Check sheet for the modelled part. Datum: model origin and axes. Units: mm. A direction names the side the tool comes from. Give positions to 0.01 mm unless a question says otherwise; leave off trailing zeros. Loops run counter-clockwise (first coordinate to the right, second up) from the corner with the lowest first, then second, coordinate; pieces in that order, holes last. Notation, with made-up numbers: (72, 40.5) -> (81, 40.5) arc R24 cw to (81, 61.5) -> close; hole circle Ø4 at (17, 33). An arc over 180 degrees is marked (long way). Write each question's results on one line, items separated by ' | '. Start each with the question number.
Item 1: Cross-section at A-A on y = 8.5. Enter the section's corners in (x, z).
Item 2: Mould release check, pull along X, two halves, no side actions. Record for faces 1 (the face through (43.6, 3, -25.9)), 2 (the face through (38.7, 1.2, -24.6)), 3 (the face through (42.15, 14, 0)): pulls with the +X half, pulls with the -X half, needs draft (parallel to the pull), parting line crosses it, or undercut.
Item 3: Access from +Z, -Z, +X, -X, +Y, -Y to the whole of each face (thin tool, end or side, straight path). Record for faces 4 (the face through (0, 13, 0)), 5 (the face through (43, 3, 26)), 6 (the face through (-36, 6, 0)), 7 (the face through (-38.56, 2.11, -28.46)).
Item 4: Scan lines: line 1 along Z through (x, y) = (40, 0.5); line 2 along X through (y, z) = (0.6, 26); line 3 along X through (y, z) = (14.7, 24.5). Record each from-to range of solid material in increasing order.
Item 5: Gauge pin test, flat ends, axial feed: pin 1 Ø1.3 at (x, z) = (36.5, -1) entering from -Y; pin 2 Ø8 at (x, z) = (-7, 2.5) entering from -Y; pin 3 Ø0.8 at (y, z) = (14, 25) entering from -X. Record the tip position at first contact, or that the pin passes through.
Item 6: Cross-section at B-B on z = 4.5. Enter the section's corners in (x, y).
from build123d import *

# Parameters (mm, degrees)
EXTRUDE_1_DEPTH          = 31
CUT_EXTRUDE_1_DEPTH      = 56.874860179
CUT_EXTRUDE_1_DEPTH_BACK = 56.874860179
SKETCH_2_W               = 42
SKETCH_2_H               = 12
CUT_EXTRUDE_3_REACH      = 57.875
SKETCH_3_R               = 1.75
SKETCH_5_R               = 1.6
CUT_EXTRUDE_5_DEPTH      = 5
CUT_EXTRUDE_8_DEPTH      = 1.6
FILLET_1_R               = 1
FILLET_7_R               = 2
CUT_EXTRUDE_9_DEPTH      = 1.8
FILLET_5_R               = 0.5
FILLET_8_R               = 1


with BuildPart() as part:
    # 草圖1 → 填料-伸長1 (new, symmetric)
    with BuildSketch(Plane.XY):
        Polygon((-44, 0), (-44, 3), (-37.15, 3), (-37.15, 13), (-42.85, 13), (-42.85, 15), (42.15, 15), (42.15, 13), (37.15, 13), (37.15, 3), (44, 3), (44, 0), (35.5, 0), (35.5, 13), (-35.5, 13), (-35.5, 0), align=None)
    extrude(amount=EXTRUDE_1_DEPTH, both=True)

    # 草圖2 → 除料-伸長1 (cut, two sides: drawn at the far end of the back side and taken through both)
    with BuildSketch(Plane(origin=(0, 0, 0), x_dir=(0, 0, -1), z_dir=(1, 0, 0)).offset(-CUT_EXTRUDE_1_DEPTH_BACK)):
        Rectangle(SKETCH_2_W, SKETCH_2_H)
    extrude(amount=CUT_EXTRUDE_1_DEPTH + CUT_EXTRUDE_1_DEPTH_BACK, mode=Mode.SUBTRACT)

    # 草圖3 → 除料-伸長3 (cut, up to next)
    with BuildSketch(Plane(origin=(0, 0, 0), x_dir=(1, 0, 0), z_dir=(0, 1, 0)), mode=Mode.PRIVATE) as cut_extrude_3_sk1:
        with Locations(Location((-40, 26, 0), (0, 0, 90))):
            Circle(SKETCH_3_R)
    cut_extrude_3_tool1 = extrude(cut_extrude_3_sk1.sketch, amount=CUT_EXTRUDE_3_REACH, mode=Mode.PRIVATE) & part.part
    # 草圖3 → 除料-伸長3 (cut, up to next)
    with BuildSketch(Plane(origin=(0, 0, 0), x_dir=(1, 0, 0), z_dir=(0, 1, 0)), mode=Mode.PRIVATE) as cut_extrude_3_sk2:
        with Locations(Location((40, 26, 0), (0, 0, 90))):
            Circle(SKETCH_3_R)
    cut_extrude_3_tool2 = extrude(cut_extrude_3_sk2.sketch, amount=CUT_EXTRUDE_3_REACH, mode=Mode.PRIVATE) & part.part
    # 草圖3 → 除料-伸長3 (cut, up to next)
    with BuildSketch(Plane(origin=(0, 0, 0), x_dir=(1, 0, 0), z_dir=(0, 1, 0)), mode=Mode.PRIVATE) as cut_extrude_3_sk3:
        with Locations(Location((40, -26, 0), (0, 0, 90))):
            Circle(SKETCH_3_R)
    cut_extrude_3_tool3 = extrude(cut_extrude_3_sk3.sketch, amount=CUT_EXTRUDE_3_REACH, mode=Mode.PRIVATE) & part.part
    # 草圖3 → 除料-伸長3 (cut, up to next)
    with BuildSketch(Plane(origin=(0, 0, 0), x_dir=(1, 0, 0), z_dir=(0, 1, 0)), mode=Mode.PRIVATE) as cut_extrude_3_sk4:
        with Locations(Location((-40, -26, 0), (0, 0, 90))):
            Circle(SKETCH_3_R)
    cut_extrude_3_tool4 = extrude(cut_extrude_3_sk4.sketch, amount=CUT_EXTRUDE_3_REACH, mode=Mode.PRIVATE) & part.part
    add(cut_extrude_3_tool1.solids().sort_by_distance((-40, 0, -26))[0], mode=Mode.SUBTRACT)
    add(cut_extrude_3_tool2.solids().sort_by_distance((40, 0, -26))[0], mode=Mode.SUBTRACT)
    add(cut_extrude_3_tool3.solids().sort_by_distance((40, 0, 26))[0], mode=Mode.SUBTRACT)
    add(cut_extrude_3_tool4.solids().sort_by_distance((-40, 0, 26))[0], mode=Mode.SUBTRACT)

    # 草圖5 → 除料-伸長5 (cut)
    with BuildSketch(Plane(origin=(0, 15, 0), x_dir=(1, 0, 0), z_dir=(0, 1, 0))):
        with Locations(Location((-39.85, 24.5, 0), (0, 0, 270))):
            Circle(SKETCH_5_R)
        with Locations(Location((-39.85, -24.5, 0), (0, 0, 270))):
            Circle(SKETCH_5_R)
        with Locations(Location((18.15, 24.5, 0), (0, 0, 270))):
            Circle(SKETCH_5_R)
        with Locations(Location((18.15, -24.5, 0), (0, 0, 270))):
            Circle(SKETCH_5_R)
    extrude(amount=-CUT_EXTRUDE_5_DEPTH, mode=Mode.SUBTRACT)

    # 草圖17 → 除料-伸長8 (cut)
    with BuildSketch(Plane.XZ.offset(-13)):
        Polygon((20.75, 22.9988893), (20.75, 26.0011107), (18.15, 27.5022214), (15.55, 26.0011107), (15.55, 22.9988893), (18.15, 21.4977786), align=None)
        Polygon((20.75, -26.0011107), (20.75, -22.9988893), (18.15, -21.4977786), (15.55, -22.9988893), (15.55, -26.0011107), (18.15, -27.5022214), align=None)
        Polygon((-39.85, 21.4977786), (-37.25, 22.9988893), (-37.25, 26.0011107), (-39.85, 27.5022214), (-42.45, 26.0011107), (-42.45, 22.9988893), align=None)
        Polygon((-39.85, -27.5022214), (-37.25, -26.0011107), (-37.25, -22.9988893), (-39.85, -21.4977786), (-42.45, -22.9988893), (-42.45, -26.0011107), align=None)
    extrude(amount=-CUT_EXTRUDE_8_DEPTH, mode=Mode.SUBTRACT)

    # 圓角1
    fillet_1_edges = [part.edges().sort_by_distance(p)[0] for p in [
        (-44, 1.5, -31),
        (-42.85, 14, -31),
        (42.15, 14, -31),
        (44, 1.5, -31),
        (44, 1.5, 31),
        (42.15, 14, 31),
        (-44, 1.5, 21),
        (-44, 1.5, -21),
        (-42.85, 14, 31),
        (44, 1.5, -21),
        (44, 1.5, 21),
        (-44, 1.5, 31),
    ]]
    fillet(fillet_1_edges, radius=FILLET_1_R)

    # 圓角7
    fillet_7_edges = [part.edges().sort_by_distance(p)[0] for p in [
        (35.5, 13, 0),
        (-35.5, 13, 0),
    ]]
    fillet(fillet_7_edges, radius=FILLET_7_R)

    # 草圖19 → 除料-伸長9 (cut)
    with BuildSketch(Plane(origin=(0, 3, 0), x_dir=(1, 0, 0), z_dir=(0, 1, 0))):
        Polygon((-40, -29.290896534), (-37.15, -27.645448267), (-37.15, -24.354551733), (-40, -22.709103466), (-42.85, -24.354551733), (-42.85, -27.645448267), align=None)
        Polygon((39.896071136, -28.850899892), (42.746071136, -27.205451625), (42.746071136, -23.91455509), (39.896071136, -22.269106823), (37.046071136, -23.91455509), (37.046071136, -27.205451625), align=None)
        Polygon((42.85, 24.354551733), (42.85, 27.645448267), (40, 29.290896534), (37.15, 27.645448267), (37.15, 24.354551733), (40, 22.709103466), align=None)
        Polygon((-40, 22.709103466), (-37.15, 24.354551733), (-37.15, 27.645448267), (-40, 29.290896534), (-42.85, 27.645448267), (-42.85, 24.354551733), align=None)
    extrude(amount=-CUT_EXTRUDE_9_DEPTH, mode=Mode.SUBTRACT)

    # 圓角5
    fillet_5_edges = [part.edges().sort_by_distance(p)[0] for p in [
        (-37.15, 3, 29.322724134),
        (37.15, 3, 29.132727491),
        (-37.15, 3, 22.677275866),
        (-37.15, 3, -29.322724134),
        (37.15, 3, -29.322724134),
        (37.15, 3, 22.427275866),
        (-37.15, 3, -22.677275866),
        (37.15, 3, -22.677275866),
    ]]
    fillet(fillet_5_edges, radius=FILLET_5_R)

    # 圓角8
    fillet_8_edges = [part.edges().sort_by_distance(p)[0] for p in [
        (37.15, 13, 0),
    ]]
    fillet(fillet_8_edges, radius=FILLET_8_R)


solid = part.part
Answer sheet:
1) outline: (-37.15, -31) -> (-35.5, -31) -> (-35.5, 31) -> (-37.15, 31) -> close; (35.5, -31) -> (37.15, -31) -> (37.15, 31) -> (35.5, 31) -> close
2) face 1: needs draft | face 2: undercut | face 3: pulls with the +X half
3) face 4: +Z, -Z, -Y | face 5: +Z, -Z, +X | face 6: +X, -X, -Y | face 7: none
4) line 1: z = -31 to -27.75, -24.25 to -21, 21 to 24.25, 27.75 to 31 | line 2: x = -44 to -41.75, -38.25 to -35.5, 35.5 to 38.25, 41.75 to 44 | line 3: x = -42.85 to -41.45, -38.25 to 16.55, 19.75 to 42.15
5) pin 1: stops at y = 6 | pin 2: stops at y = 13 | pin 3: stops at x = -42.85
6) outline: (-42.85, 13) -> (-37.15, 13) -> (-37.15, 6) -> (-35.5, 6) -> (-35.5, 11) arc R2 cw to (-33.5, 13) -> (33.5, 13) arc R2 cw to (35.5, 11) -> (35.5, 6) -> (37.15, 6) -> (37.15, 12) arc R1 cw to (38.15, 13) -> (42.15, 13) -> (42.15, 15) -> (-42.85, 15) -> close
